```python
from build123d import *

# Parameters (mm, degrees)
F3_R      = 1.85
F4_DEPTH  = 7
F5_R      = 1.2
F6_DEPTH  = 2
F8_DEPTH  = 4.5
F9_R      = 1
F10_R     = 1.2
F11_DEPTH = 4.5
F12_R     = 5
F13_R     = 14
F13_R_2   = 11
F14_DEPTH = 0.2


with BuildPart() as f1:
    # F0 (on Top) → F1 (revolve)
    with BuildSketch(Plane.XY):
        with BuildLine():
            Line((0, 9), (0, 0))
            Line((0, 0), (11, 0))
            Line((11, 0), (11, 4))
            Line((11, 4), (10.5, 7))
            ThreePointArc((10.5, 7), (10.0017468007, 7.1915925315), (9.5, 7.3738398822))
            Line((9.5, 7.3738398822), (9.5, 6.5449972332))
            Line((9.5, 6.5449972332), (9, 6.5449972332))
            Line((9, 6.5449972332), (9, 7.5449972332))
            ThreePointArc((9, 7.5449972332), (4.5584271698, 8.6339031037), (0, 9))
        make_face()
    revolve(axis=Axis((0, 4.5, 0), (0, 1, 0)))

    # F3 (on offset) → F4 (cut)
    with BuildSketch(Plane.XZ.offset(-9)):
        with Locations((6.65, 4.625)):
            Circle(F3_R)
    extrude(amount=F4_DEPTH, mode=Mode.SUBTRACT)

    # F5 (on face) → F6 (cut, through all)
    with BuildSketch(Plane(origin=(0, 2, 0), x_dir=(-1, 0, 0), z_dir=(0, 1, 0))):
        with Locations((-6.65, 4.625)):
            Circle(F5_R)
    extrude(amount=-F6_DEPTH, mode=Mode.SUBTRACT)

    # F7 (on offset) → F8 (cut)
    with BuildSketch(Plane.XZ.offset(-9)):
        with BuildLine():
            Line((4.9918584287, -4.0461524227), (-3.38657071, 10.4657125331))
            ThreePointArc((-3.38657071, 10.4657125331), (-8.661662033, 6.780531751), (-10.9726648996, 0.775))
            Line((-10.9726648996, 0.775), (-3.1032576969, 0.775))
            Line((-3.1032576969, 0.775), (1.0081415713, -6.3461524227))
            Line((1.0081415713, -6.3461524227), (4.9918584287, -4.0461524227))
        make_face()
    extrude(amount=F8_DEPTH, mode=Mode.SUBTRACT)

    # F9
    f9_edges = [f1.edges().sort_by_distance(p)[0] for p in [
        (4.991858, 6.383907, -4.046152),
        (1.008142, 6.383907, -6.346152),
    ]]
    fillet(f9_edges, radius=F9_R)

    # F10 (on face) → F11 (cut, through all)
    with BuildSketch(Plane(origin=(0, 4.5, 0), x_dir=(-1, 0, 0), z_dir=(0, 1, 0))):
        with Locations((6.65, 4.625)):
            Circle(F10_R)
    extrude(amount=-F11_DEPTH, mode=Mode.SUBTRACT)

    # F12
    f12_edges = [f1.edges().sort_by_distance(p)[0] for p in [
        (-3.103258, 6.66017, 0.775),
    ]]
    fillet(f12_edges, radius=F12_R)

    # F13 (on face) → F14 (join)
    with BuildSketch(Plane.XZ):
        Circle(F13_R)
        Circle(F13_R_2, mode=Mode.SUBTRACT)
    extrude(amount=-F14_DEPTH)


solid = f1.part
```
Geometry: final body of the model. Coordinates: model frame, mm. A direction names the side the tool comes from. Coordinates: 2 decimals unless noted, no trailing zeros. Order: outer loops, then holes, each group sorted by start corner. A loop starts at its lowest first (then second) coordinate and runs counter-clockwise, first axis right, second up. Notation, with made-up numbers: (-23, 70.25) -> (24, 70.25) arc R20 ccw to (24, 78.25) -> close; hole circle Ø5 at (62, 50). An arc over 180 degrees is marked (long way). Use CSV: the item, a comma, the result in double quotes.
1) Section D-D on x = -11.75. Output: boundary loops of the cut face in (y, z).
Findings:
outline,"(0, -7.61) -> (0.2, -7.61) -> (0.2, 7.61) -> (0, 7.61) -> close"
2) Mould query, pull axis Z, two halves, no side actions, for faces 4 (the conical face through (10.04, 6.85, -3.16)), 5 (the cylindrical face through (4.6, 6.5, -3.9)), 6 (the flat face through (6.2, 0.2, -9.3)), 7 (the cylindrical face through (-3.458, 6.672, 0.087)). Classes: +Z half, -Z half, draft (parallel to the pull), parting line (faces both ways), or undercut.
Findings:
face 4,"parting line"
face 5,"undercut"
face 6,"draft"
face 7,"undercut"
3) Section A-A on y = 5. Output: boundary loops of the cut face in (x, z) (3 decimals), then the cut area to 3 significant figures.
Findings:
outline,"(-10.806, 0.775) arc R10.833 ccw (long way) to (-3.301, 10.318) -> (4.492, -3.18) arc R1 cw to (4.126, -4.546) -> (1.874, -5.846) arc R1 cw to (0.508, -5.48) -> (-1.66, -1.725) arc R5 ccw to (-5.99, 0.775) -> close; hole circle Ø3.7 at (6.65, 4.625)"
area,"248 mm^2"
4) Line query: line 1 (X direction, y = 6.75, z = -4); line 2 (Y direction, x = 5.75, z = -11.5); line 3 (Z direction, x = 6.65, y = 1.55) (3 decimals). Output: solid intervals per line, ascending.
Findings:
line 1,"x = -9.75 to -8.62, -8.06 to -0.35, 4.57 to 8.06, 8.62 to 9.75"
line 2,"y = 0 to 0.2"
line 3,"z = -8.762 to 3.425, 5.825 to 8.762"
5) Pin query (flat end, axial travel): pin 1 Ø1.2 at (x, y) = (-9, 6) entering from +Z (3 decimals); pin 2 Ø2 at (y, z) = (6.5, -9) entering from -X; pin 3 Ø2 at (x, z) = (-6.65, 4.625) entering from -Y; pin 4 Ø1 at (x, y) = (-1.5, 5) entering from +Z. Return the tip coordinate at first contact, or that it passes through.
Findings:
pin 1,"stops at z = 0.775"
pin 2,"stops at x = -6.96"
pin 3,"passes through"
pin 4,"stops at z = 10.83"
6) Access query for faces 1 (the flat face through (-8, 6, 0.775)), 2 (the cylindrical face through (-2.38, 2.13, 10.74)), 3 (the flat face through (0, 0, 0)). Directions: +Z, -Z, +X, -X, +Y, -Y. A direction counts if a zero-diameter tool reaches every point of the face in a straight line with its end or side. Return the directions, or none.
Findings:
face 1,"+Z, -X, +Y"
face 2,"+Y"
face 3,"+Z, -Z, +X, -X, -Y"
